Input: dimensioned drawing with shaded views. Units: mm. Origin: part minimum x, y, z. A direction names the side the tool comes from. Coordinates: 2 decimals unless noted, no trailing zeros. Order: outer loops, then holes, each group sorted by start corner. A loop starts at its lowest first (then second) coordinate and runs counter-clockwise, first axis right, second up. Notation, with made-up numbers: (-25, 56.5) -> (-19, 56.5) arc R24 ccw to (-19, 87.5) -> close; hole circle Ø10 at (40.5, 69.5). An arc over 180 degrees is marked (long way). Write item = value, one per line. Start each with the question number.
Item 1: Section query C-C (z = 37). Output: boundary loops of the cut face in (x, y) (1 decimal).
Item 2: Set-up query: the marked faces 1 and 2. Return all of +Z, -Z, +X, -X, +Y, -Y with unobstructed straight access to the full face (end or side cutting, diameter ignored); none if empty.
Item 3: Ray query, line 1 along Y through (x, z) = (5, 37.5); line 2 along Z through (x, y) = (57.5, 22.5) (1 decimal); line 3 along X through (y, z) = (22, 46) (1 decimal). Return the intervals inside material, ascending. Write a range as [from, to].
Item 4: Contact query for flat-ended pins moving along their axis: pin 1 (12 mm diameter, centred on y = 57, z = 19, fed in from -X); pin 2 (12 mm diameter, centred on x = 26.5, y = 17, fed in from +Z); pin 3 (12 mm diameter, centred on x = 40.5, z = 42, fed in from +Y); pin 4 (3 mm diameter, centred on x = 78, z = 31.5, fed in from -Y). Output: stop coordinate, or through.
Item 5: Section query D-D (x = 64). Output: boundary loops of the cut face in (y, z).
Item 6: Section query B-B (y = 43). Output: boundary loops of the cut face in (x, z) (1 decimal), then the cut area to 3 significant figures.
Item 7: Section query A-A (x = 40). Output: boundary loops of the cut face in (y, z) (1 decimal), then the cut area to 3 significant figures.
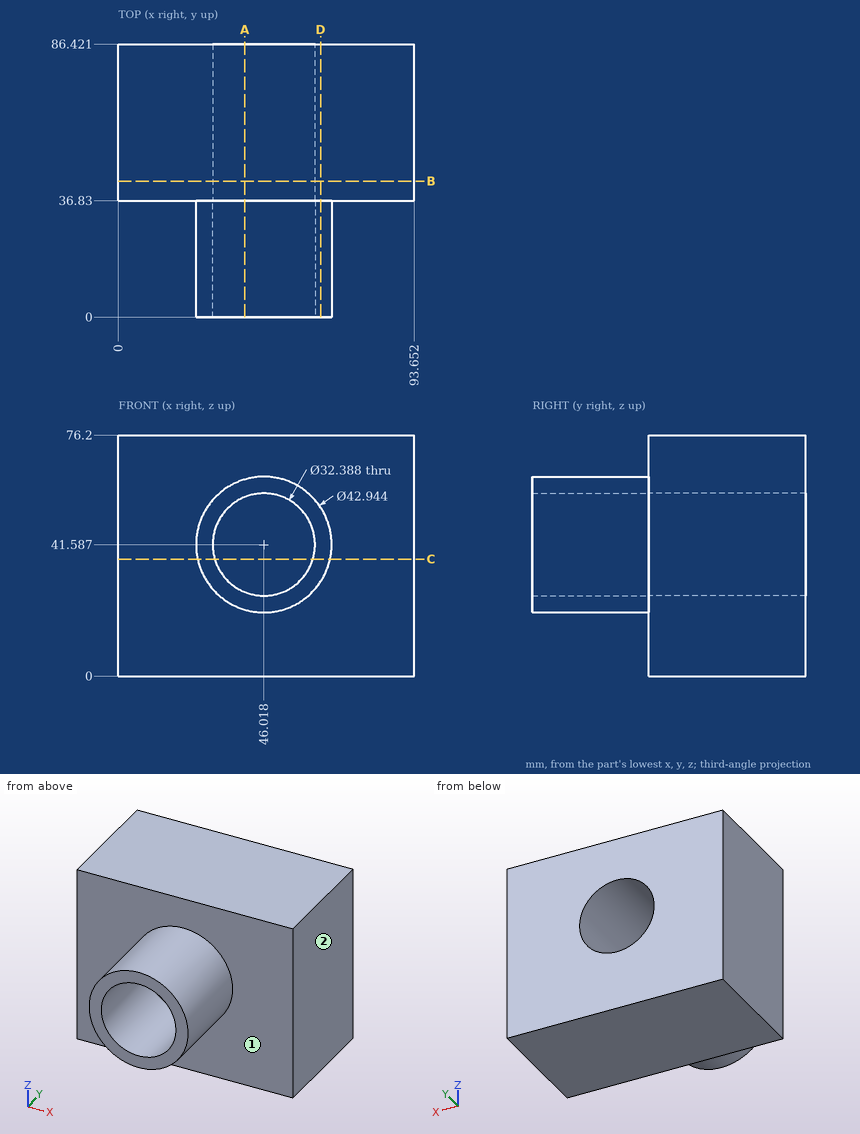
Computed:
q1.outline = (0, 36.8) -> (25, 36.8) -> (25, 0) -> (30.5, 0) -> (30.5, 86.4) -> (0, 86.4) -> close; (61.5, 0) -> (67, 0) -> (67, 36.8) -> (93.7, 36.8) -> (93.7, 86.4) -> (61.5, 86.4) -> close
q2.face_1 = -Y
q2.face_2 = +Z, -Z, +X, +Y, -Y
q3.line_1 = [36.83, 86.42]
q3.line_2 = [23.4, 30.2], [53, 59.7]
q3.line_3 = [25, 30.4], [61.6, 67]
q4.pin_1 = 0
q4.pin_2 = 58.27
q4.pin_3 = through
q4.pin_4 = 36.83
q5.outline = (0, 29.85) -> (36.83, 29.85) -> (36.83, 0) -> (86.42, 0) -> (86.42, 76.2) -> (36.83, 76.2) -> (36.83, 53.32) -> (0, 53.32) -> close
q6.outline = (0, 0) -> (93.7, 0) -> (93.7, 76.2) -> (0, 76.2) -> close; hole circle Ø32.4 at (46, 41.6)
q6.area = 6,310 mm^2
q7.outline = (0, 21) -> (36.8, 21) -> (36.8, 0) -> (86.4, 0) -> (86.4, 26.6) -> (0, 26.6) -> close; (0, 56.6) -> (86.4, 56.6) -> (86.4, 76.2) -> (36.8, 76.2) -> (36.8, 62.2) -> (0, 62.2) -> close
q7.area = 2,700 mm^2
